Part model, mm, in its own coordinate system. Face numbers are marked on the shaded views. Give positions to 0.01 mm unless a question says otherwise; leave off trailing zeros. Loops run counter-clockwise (first coordinate to the right, second up) from the corner with the lowest first, then second, coordinate; pieces in that order, holes last. Notation, with made-up numbers: M 28.5,-14.5 L 37.5,-14.5 A30 cw 37.5,22.5 Z; hole C -31.5,82 d7. An arc over 180 degrees is marked long. Answer in a Markdown table with one row per item.
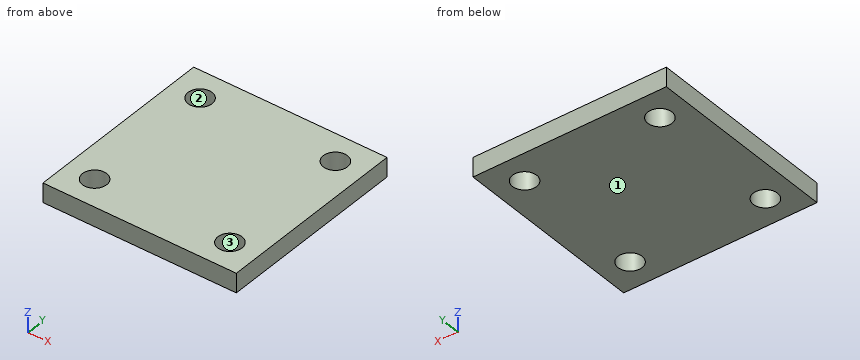
from build123d import *

# Parameters (mm, degrees)
F0_W     = 20
F0_H     = 20
F1_DEPTH = 2
F3_D     = 2.5


with BuildPart() as f1:
    # F0 (on Top) → F1 (new body)
    with BuildSketch(Plane.XY):
        Rectangle(F0_W, F0_H)
    extrude(amount=-F1_DEPTH)

    # F3 (through all)
    with Locations(Plane.XY):
        with Locations((-7, 7), (7, 7), (-7, -7), (7, -7)):
            Hole(F3_D / 2)


solid = f1.part
(1) Pull direction X, two halves, no side cores. Call the marked faces 1, 2 and 3: +X half, -X half, draft (parallel to the pull), parting line (faces both ways), or undercut.
Recorded:
| item | result |
|---|---|
| face 1 | draft |
| face 2 | undercut |
| face 3 | undercut |
(2) Saw through at A-A (y = -7). Write the cut outline in (x, z).
Recorded:
| item | result |
|---|---|
| outline | M -10,-2 L -8.25,-2 L -8.25,0 L -10,0 Z; M -5.75,-2 L 5.75,-2 L 5.75,0 L -5.75,0 Z; M 8.25,-2 L 10,-2 L 10,0 L 8.25,0 Z |
(3) Drill centre lines: line 1 along Y through (x, z) = (-7, -1.6); line 2 along Y through (x, z) = (7.5, -0.1). Where is each one in solid material? Low to high.
Recorded:
| item | result |
|---|---|
| line 1 | y = -10 to -8.25, -5.75 to 5.75, 8.25 to 10 |
| line 2 | y = -10 to -8.15, -5.85 to 5.85, 8.15 to 10 |
(4) Saw through at C-C (z = -0.25). Write the cut outline in (x, y).
Recorded:
| item | result |
|---|---|
| outline | M -10,-10 L 10,-10 L 10,10 L -10,10 Z; hole C -7,-7 d2.5; hole C -7,7 d2.5; hole C 7,-7 d2.5; hole C 7,7 d2.5 |
